Solid Edge part; units mm, degrees
sketch "Sketch1" plane through (0, 0, 0) normal (0, 0, 1) x (1, 0, 0)
  line L0 (0, 0) -> (0, 254)
  line L1 (0, 254) -> (203.2, 254)
  line L2 (203.2, 254) -> (203.2, 0)
  line L3 (203.2, 0) -> (0, 0)
  dimension "D1" = 203.2
extrude "Protrusion1" add sketch "Sketch1" along normal blind 3.175
hole "Hole_1" at (158.75, 139.7, 3.175) direction (0, 0, -1) diameter 6.35 end up to next
hole "Hole1" at (158.75, 25.4, 3.175) direction (0, 0, -1) diameter 6.35 end up to next
hole "Hole2" at (44.45, 25.4, 3.175) direction (0, 0, -1) diameter 6.35 end up to next
hole "Hole3" at (44.45, 139.7, 3.175) direction (0, 0, -1) diameter 6.35 end up to next
fillet "Round_1" radius 12.7 4 edges at (0, 0, 1.5875) (203.2, 0, 1.5875) (203.2, 254, 1.5875) (0, 254, 1.5875)
properties part number "CHAS-05" material "Acrylic, high impact grade"
Part model, mm, in its own coordinate system. Coordinates: 2 decimals unless noted, no trailing zeros. Order: outer loops, then holes, each group sorted by start corner. A loop starts at its lowest first (then second) coordinate and runs counter-clockwise, first axis right, second up. Notation, with made-up numbers: M 35,42 L 41,42 A10 cw 41,59 Z; hole C 41,12 d4. An arc over 180 degrees is marked long. One line per question, with ' | ' between items.
Q1. Two-plate mould, pull along X, no slides. Class faces 1 (the face through (161.9, 140.1, 1.6)), 2 (the face through (199.38, 3.62, 1.61)), 3 (the face through (103, 129, 3.175)), 4 (the face through (3.62, 3.82, 1.61)): +X half, -X half, draft (parallel to the pull), parting line (faces both ways), or undercut.
A:
face 1: undercut | face 2: +X half | face 3: draft | face 4: -X half
Q2. Drill centre lines: line 1 (X direction, y = 139.7, z = 1.9) (3 decimals); line 2 (Y direction, x = 158.75, z = 1.1) (3 decimals); line 3 (X direction, y = 11, z = 1.8). Where is each one in solid material? Low to high.
A:
line 1: x = 0 to 41.275, 47.625 to 155.575, 161.925 to 203.2 | line 2: y = 0 to 22.225, 28.575 to 136.525, 142.875 to 254 | line 3: x = 0.11 to 203.09
Q3. Slice it at A-A (x = 44.45). Give the cut face in (y, z) (3 decimals).
A:
outline: M 0,0 L 22.225,0 L 22.225,3.175 L 0,3.175 Z; M 28.575,0 L 136.525,0 L 136.525,3.175 L 28.575,3.175 Z; M 142.875,0 L 254,0 L 254,3.175 L 142.875,3.175 Z
Q4. Pin check, flat tip, straight feed: P1, Ø8.5, axis at x = 158.75, y = 25.4, coming from the -Z side. Stop position of the tip, or through.
A:
P1: stops at z = 0
Q5. Slice it at B-B (y = 139.7). Give the cut face in (x, z) (3 decimals).
A:
outline: M 0,0 L 41.275,0 L 41.275,3.175 L 0,3.175 Z; M 47.625,0 L 155.575,0 L 155.575,3.175 L 47.625,3.175 Z; M 161.925,0 L 203.2,0 L 203.2,3.175 L 161.925,3.175 Z
